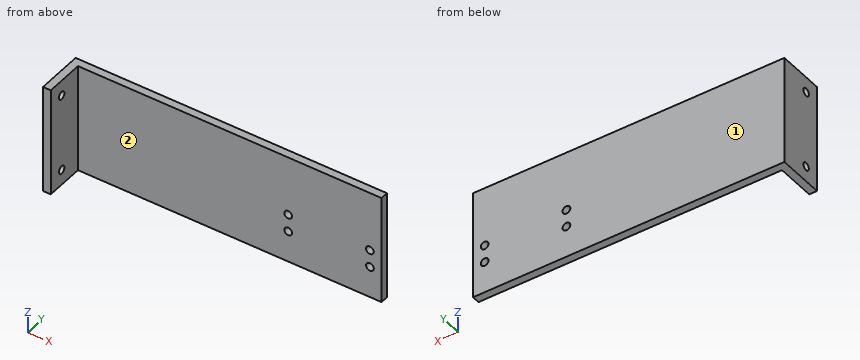
```python
from build123d import *

# Parameters (mm, degrees)
F0_W     = 254
F0_H     = 88.9
F1_DEPTH = 6.35
F3_D     = 6.35
F4_W     = 6.35
F4_H     = 88.9
F5_DEPTH = 31.75
F7_D     = 6.35


with BuildPart() as f1:
    # F0 (on Front) → F1 (new body)
    with BuildSketch(Plane.XZ):
        with Locations((97.875736, -13.176627)):
            Rectangle(F0_W, F0_H)
    extrude(amount=F1_DEPTH)

    # F3 (through all)
    with Locations(Plane.XZ.offset(6.35)):
        with Locations((148.675736, -17.621627), (215.376136, -17.621627), (215.376136, -31.896427), (148.675736, -31.896427)):
            Hole(F3_D / 2)

    # F4 (on face) → F5 (join)
    with BuildSketch(Plane.XZ.offset(6.35)):
        with Locations((-25.949264, -13.176627)):
            Rectangle(F4_W, F4_H)
    extrude(amount=F5_DEPTH)

    # F7 (through all)
    with Locations(Plane.YZ.offset(-22.774264)):
        with Locations((-25.4, -44.926627), (-25.4, 18.573373)):
            Hole(F7_D / 2)


solid = f1.part
```
Input: part model. Units: mm. Frame: model coordinates. Face numbers are marked on the shaded views. A direction names the side the tool comes from. Coordinates: 2 decimals unless noted, no trailing zeros. Order: outer loops, then holes, each group sorted by start corner. A loop starts at its lowest first (then second) coordinate and runs counter-clockwise, first axis right, second up. Notation, with made-up numbers: (-12.5, 55) - (33.5, 55) arc R16 ccw to (33.5, 75) - close; hole circle Ø2 at (16.25, 47.25). An arc over 180 degrees is marked (long way). Put each result on its own line as item: value.
1. Line query: line 1 along X through (y, z) = (-22, -48); line 2 along Y through (x, z) = (154, 0). Output: solid intervals per line, ascending.
Report:
line 1: x = -29.12 to -22.77
line 2: y = -6.35 to 0
2. Contact query for flat-ended pins moving along their axis: pin 1 Ø10 at (x, z) = (163, -11.5) entering from -Y; pin 2 Ø8 at (y, z) = (-25, -38.5) entering from +X. Output: stop coordinate, or through.
Report:
pin 1: stops at y = -6.35
pin 2: stops at x = -22.77
3. Cut plane B-B on z = 4.5. Return the cut outline in (x, y).
Report:
outline: (-29.12, -38.1) - (-22.77, -38.1) - (-22.77, -6.35) - (224.88, -6.35) - (224.88, 0) - (-29.12, 0) - close
4. Reachability of the marked faces 1 and 2 from +Z, -Z, +X, -X, +Y, -Y: full face, straight path, thin tool, end or side. Return the list, or none.
Report:
face 1: +Z, -Z, +X, -X, +Y
face 2: +Z, -Z, +X, -Y
5. Cut plane A-A on y = -25.4. Return the cut outline in (x, z), then the cut area to 3 significant figures.
Report:
outline: (-29.12, -57.63) - (-22.77, -57.63) - (-22.77, -48.1) - (-29.12, -48.1) - close; (-29.12, -41.75) - (-22.77, -41.75) - (-22.77, 15.4) - (-29.12, 15.4) - close; (-29.12, 21.75) - (-22.77, 21.75) - (-22.77, 31.27) - (-29.12, 31.27) - close
area: 484 mm2
6. Cut plane C-C on x = 195. Return the cut outline in (y, z), then the cut area to 3 significant figures.
Report:
outline: (-6.35, -57.63) - (0, -57.63) - (0, 31.27) - (-6.35, 31.27) - close
area: 565 mm2
